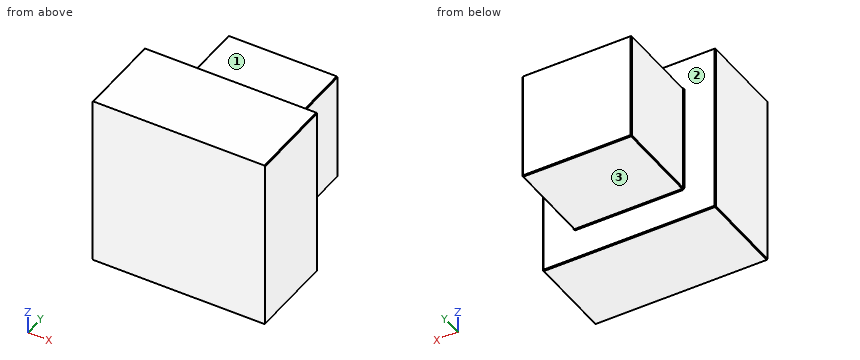
```python
from build123d import *

# Parameters (mm, degrees)
ESQUISSE1_W        = 6
ESQUISSE1_H        = 6
BOSS_EXTRU_1_DEPTH = 3
ESQUISSE2_W        = 3.8
ESQUISSE2_H        = 3.8
BOSS_EXTRU_2_DEPTH = 3
CHANFREIN1_SIZE    = 0.03


with BuildPart() as part:
    # Esquisse1 → Boss.-Extru.1 (new body)
    with BuildSketch(Plane(origin=(0, 0, 0), x_dir=(1, 0, 0), z_dir=(0, 1, 0))):
        Rectangle(ESQUISSE1_W, ESQUISSE1_H)
    extrude(amount=BOSS_EXTRU_1_DEPTH)

    # Esquisse2 → Boss.-Extru.2 (add)
    with BuildSketch(Plane(origin=(0, 3, 0), x_dir=(1, 0, 0), z_dir=(0, 1, 0))):
        Rectangle(ESQUISSE2_W, ESQUISSE2_H)
    extrude(amount=BOSS_EXTRU_2_DEPTH)

    # Chanfrein1
    chanfrein1_edges = [part.edges().sort_by_distance(p)[0] for p in [
        (-3, 3, 0),
        (1.9, 3, 0),
        (1.9, 4.5, 1.9),
        (0, 3, 3),
        (0, 3, -1.9),
        (1.9, 4.5, -1.9),
        (-1.9, 3, 0),
        (-1.9, 4.5, -1.9),
        (0, 3, 1.9),
        (-1.9, 4.5, 1.9),
        (1.9, 6, 0),
        (0, 6, -1.9),
        (-1.9, 6, 0),
        (0, 6, 1.9),
        (3, 3, 0),
        (3, 1.5, 3),
        (-3, 1.5, 3),
        (-3, 1.5, -3),
        (3, 1.5, -3),
        (0, 3, -3),
    ]]
    chamfer(chanfrein1_edges, length=CHANFREIN1_SIZE)


solid = part.part
```
Geometry check sheet. Reference: the model listing, model coordinates, mm. Face numbers are marked on the shaded views. A direction names the side the tool comes from. Round coordinates to 2 decimals unless told otherwise and drop trailing zeros. Loops run counter-clockwise (first coordinate to the right, second up) from the corner with the lowest first, then second, coordinate; pieces in that order, holes last. Notation, with made-up numbers: (86.25, -35.75) - (93.25, -35.75) arc R32 cw to (93.25, -6.75) - close; hole circle Ø7 at (-1.5, 56). An arc over 180 degrees is marked (long way). Write item = value, one per line. Start each with the question number.
1. Depth check by flat-ended pin: pin 1 (1.5 mm diameter, centred on y = 4, z = 1, fed in from +X); pin 2 (1.5 mm diameter, centred on x = 0, y = 5, fed in from -Z); pin 3 (3 mm diameter, centred on x = 0, y = 5, fed in from +Z). Enter the tip coordinate at first touch or a pass-through.
2. Section check B-B on z = -1.5. Enter the section's corners in (x, y), then the cut area to 3 significant figures.
3. Thickness scan on line 1 (Y direction, x = -2.5, z = 1); line 2 (X direction, y = 5.75, z = 1). Record the ranges inside material, lowest first.
4. Section check C-C on y = 3.5. Enter the section's corners in (x, z).
5. Section check A-A on x = 1.5. Enter the section's corners in (y, z).
6. Section check D-D on z = 2.25. Enter the section's corners in (x, y).
7. Set-up check for the marked faces 1, 2 and 3: record each of +Z, -Z, +X, -X, +Y, -Y from which the full face is reachable in a straight line by a thin tool's end or side.
Working result:
q1.pin_1 = 1.9
q1.pin_2 = -1.9
q1.pin_3 = 1.9
q2.outline = (-3, 0) - (3, 0) - (3, 2.97) - (2.97, 3) - (1.93, 3) - (1.9, 3.03) - (1.9, 5.97) - (1.87, 6) - (-1.87, 6) - (-1.9, 5.97) - (-1.9, 3.03) - (-1.93, 3) - (-2.97, 3) - (-3, 2.97) - close
q2.area = 29.4 mm^2
q3.line_1 = 0 to 3
q3.line_2 = -1.9 to 1.9
q4.outline = (-1.9, -1.87) - (-1.87, -1.9) - (1.87, -1.9) - (1.9, -1.87) - (1.9, 1.87) - (1.87, 1.9) - (-1.87, 1.9) - (-1.9, 1.87) - close
q5.outline = (0, -3) - (2.97, -3) - (3, -2.97) - (3, -1.93) - (3.03, -1.9) - (5.97, -1.9) - (6, -1.87) - (6, 1.87) - (5.97, 1.9) - (3.03, 1.9) - (3, 1.93) - (3, 2.97) - (2.97, 3) - (0, 3) - close
q6.outline = (-3, 0) - (3, 0) - (3, 2.97) - (2.97, 3) - (-2.97, 3) - (-3, 2.97) - close
q7.face_1 = +Z, +X, -X, +Y
q7.face_2 = +Y
q7.face_3 = -Z, +X, -X, +Y
